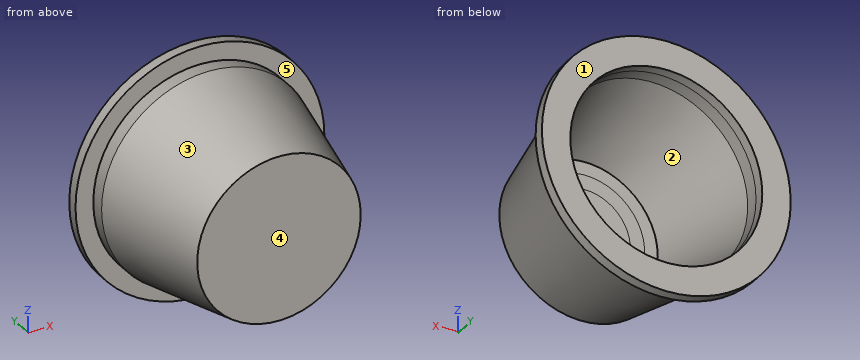
from build123d import *

# Parameters (mm, degrees)
F0_R      = 30
F0_R_2    = 27
F1_DEPTH  = 4
F4_R      = 30
F3_R      = 23
F7_R      = 20
F6_R      = 27
F9_R      = 22.403667
F9_R_2    = 12.693191
F10_DEPTH = 2
F11_R     = 35
F11_R_2   = 27
F12_DEPTH = 3
F13_R     = 16.737404
F14_DEPTH = 2


with BuildPart() as f1:
    # F0 (on Front) → F1 (new body)
    with BuildSketch(Plane.XZ):
        Circle(F0_R)
        Circle(F0_R_2, mode=Mode.SUBTRACT)
    extrude(amount=F1_DEPTH)

    # F4 (on face) → F5 section 0
    with BuildSketch(Plane.XZ.offset(4)):
        Circle(F4_R)
    # F3 (on offset) → F5 section 1
    with BuildSketch(Plane.XZ.offset(38)):
        Circle(F3_R)
    loft()

    # F7 (on face) → F8 section 0
    with BuildSketch(Plane.XZ.offset(38)):
        Circle(F7_R)
    # F6 (on face) → F8 section 1
    with BuildSketch(Plane(origin=(0, -4, 0), x_dir=(-1, 0, 0), z_dir=(0, 1, 0))):
        Circle(F6_R)
    loft(mode=Mode.SUBTRACT)

    # F9 (on face) → F10 (join)
    with BuildSketch(Plane.XZ.offset(38)):
        Circle(F9_R)
        Circle(F9_R_2, mode=Mode.SUBTRACT)
    extrude(amount=-F10_DEPTH)

    # F11 (on face) → F12 (join)
    with BuildSketch(Plane(origin=(0, 0, 0), x_dir=(-1, 0, 0), z_dir=(0, 1, 0))):
        Circle(F11_R)
        Circle(F11_R_2, mode=Mode.SUBTRACT)
    extrude(amount=F12_DEPTH)

    # F13 (on face) → F14 (join)
    with BuildSketch(Plane.XZ.offset(38)):
        Circle(F13_R)
    extrude(amount=-F14_DEPTH)


solid = f1.part
Geometry: final body of the model. Coordinates: model frame, mm. Face numbers are marked on the shaded views. A direction names the side the tool comes from. Give positions to 0.01 mm unless a question says otherwise; leave off trailing zeros. Order: outer loops, then holes, each group sorted by start corner. A loop starts at its lowest first (then second) coordinate and runs counter-clockwise, first axis right, second up. Notation, with made-up numbers: (-7.5, 45) -> (11.5, 45) arc R21 ccw to (11.5, 76) -> close; hole circle Ø2 at (23, 29.25). An arc over 180 degrees is marked (long way). Answer as a JSON object with one key per item and string values.
Q1. Section C-C (y = -20.5). Output: boundary loops of the cut face in (x, z), plus the area to 3 significant figures.
Entries:
{"outline": "circle Ø53.21 at (0, 0); hole circle Ø47.21 at (0, 0)", "area": "473 mm^2"}
Q2. Section B-B (y = -2.5). Output: boundary loops of the cut face in (x, z).
Entries:
{"outline": "circle Ø60 at (0, 0); hole circle Ø54 at (0, 0)"}
Q3. Section A-A (x = 0). Output: boundary loops of the cut face in (y, z).
Entries:
{"outline": "(-38, -23) -> (-4, -30) -> (0, -30) -> (0, -35) -> (3, -35) -> (3, -27) -> (-4, -27) -> (-36, -20.41) -> (-36, 20.41) -> (-4, 27) -> (3, 27) -> (3, 35) -> (0, 35) -> (0, 30) -> (-4, 30) -> (-38, 23) -> close"}
Q4. Draft query along Z for the marked faces 1, 2 and 3. Return one class per face: released by +Z, released by -Z, zero draft, split by the parting line, or undercut.
Entries:
{"face 1": "zero draft", "face 2": "undercut", "face 3": "split by the parting line"}
Q5. First-contact query: pin 1 (5 mm diameter, centred on y = -23, z = -17.5, fed in from -X); pin 2 (5 mm diameter, centred on x = 8.5, y = -21, fed in from -Z); pin 3 (1 mm diameter, centred on y = -9, z = -4.5, fed in from +X). Flat tips, straight axial feed; report the tip coordinate or a pass-through.
Entries:
{"pin 1": "stops at x = -21.45", "pin 2": "stops at z = -26.01", "pin 3": "stops at x = 28.75"}
Q6. Access query for the marked faces 4 and 5. Directions: +Z, -Z, +X, -X, +Y, -Y. A direction counts if a zero-diameter tool reaches every point of the face in a straight line with its end or side. Return the directions, or none.
Entries:
{"face 4": "+Z, -Z, +X, -X, -Y", "face 5": "-Y"}
Q7. Material intervals for probe 1 along Z at (x, y) = (0, 2); probe 2 along Z at (x, y) = (0, -1.1); probe 3 along X at (y, z) = (-34, 1), sorted ascending.
Entries:
{"probe 1": "z = -35 to -27, 27 to 35", "probe 2": "z = -30 to -27, 27 to 30", "probe 3": "x = -23.8 to -20.8, 20.8 to 23.8"}
